from build123d import *

# Parameters (mm, degrees)
CHAMFER_1_SIZE      = 1
CUT_EXTRUDE_1_DEPTH = 37.221540553
SKETCH_3_R          = 10
EXTRUDE_1_DEPTH     = 15
CHAMFER_2_SIZE      = 0.5
SKETCH_7_W          = 0.7
SKETCH_7_H          = 1.1


with BuildPart() as part:
    # 草图1 → 旋转1 (revolve)
    with BuildSketch(Plane.XY, mode=Mode.PRIVATE) as revolve_1_sk:
        Polygon((0, 0), (10, 0), (10, 1.992934229), (10, 22), (12, 22), (12, 32), (9, 32), (9, 52), (0, 52), align=None)
    revolve(revolve_1_sk.sketch.rotate(Axis((0, 0, 0), (0, 1, 0)), 90), axis=Axis((0, 0, 0), (0, 1, 0)))

    # 倒角1
    chamfer_1_edges = [part.edges().sort_by_distance(p)[0] for p in [
        (0, 52, 9),
    ]]
    chamfer(chamfer_1_edges, length=CHAMFER_1_SIZE)

    # 草图2 → 切除-拉伸1 (cut, through all)
    with BuildSketch(Plane(origin=(0, 32, 0), x_dir=(1, 0, 0), z_dir=(0, 1, 0))):
        with BuildLine():
            Line((-11, -4.795831523), (-11, 4.795831523))
            ThreePointArc((-11, 4.795831523), (-12, 0), (-11, -4.795831523))
        make_face()
        with BuildLine():
            ThreePointArc((12, 0), (11.747340124, 2.449489743), (11, 4.795831523))
            Line((11, 4.795831523), (11, -4.795831523))
            ThreePointArc((11, -4.795831523), (11.747340124, -2.449489743), (12, 0))
        make_face()
    extrude(amount=-CUT_EXTRUDE_1_DEPTH, mode=Mode.SUBTRACT)

    # 草图3 → 凸台-拉伸1 (add)
    with BuildSketch(Plane.XZ):
        with Locations(Location((0, 0, 0), (0, 0, 270))):
            Circle(SKETCH_3_R)
    extrude(amount=EXTRUDE_1_DEPTH)

    # 倒角2
    chamfer_2_edges = [part.edges().sort_by_distance(p)[0] for p in [
        (0, -15, 10),
    ]]
    chamfer(chamfer_2_edges, length=CHAMFER_2_SIZE)

    # 草图7 → 切除-旋转1 (revolve, cut)
    with BuildSketch(Plane(origin=(0, 0, 0), x_dir=(0, 0, -1), z_dir=(1, 0, 0))):
        with Locations((9.65, -12.05)):
            Rectangle(SKETCH_7_W, SKETCH_7_H)
    revolve(axis=Axis((0, 52, 0), (0, -1, 0)), mode=Mode.SUBTRACT)


solid = part.part
Verification items for the finished model (mm, model axes). A direction names the side the tool comes from. Give positions to 0.01 mm unless a question says otherwise; leave off trailing zeros. Loops run counter-clockwise (first coordinate to the right, second up) from the corner with the lowest first, then second, coordinate; pieces in that order, holes last.
1) Thickness scan on line 1 along Y through (x, z) = (-9, -2.75); line 2 along Y through (x, z) = (3.5, -10); line 3 along Y through (x, z) = (7.5, -6.5). Record the ranges inside material, lowest first.
2) Depth check by flat-ended pin: pin 1 Ø6 at (x, y) = (5, 7.5) entering from -Z; pin 2 Ø2 at (x, y) = (1, 41.5) entering from -Z; pin 3 Ø1.5 at (x, y) = (-3, 13) entering from +Z. Enter the tip coordinate at first touch or a pass-through.
3) Set-up check for faces 1 (the cylindrical face through (-9.76, 5.48, 2.17)), 2 (the cylindrical face through (7.84, -12.04, -5)), 3 (the flat face through (-7, 32, 6)): record each of +Z, -Z, +X, -X, +Y, -Y from which the full face is reachable in a straight line by a thin tool's end or side.
4) Sectioned sample at D-D, the plane y = 5. Enter the section's corners in (x, z), then the cut area to 3 significant figures.
5) Sectioned sample at A-A, the plane z = 0. Enter the section's corners in (x, y), then the cut area to 3 significant figures.
6) Sectioned sample at B-B, the plane x = 0. Enter the section's corners in (y, z).
7) Sectioned sample at C-C, the plane y = 24. Enter the section's corners in (x, z), then the cut area to 3 significant figures.
8) Draft check along Y on faces 4 (the flat face through (-9, -12.6, 3)), 5 (the flat face through (11, 27, 0)), 6 (the flat face through (0, -15, 0)), 7 (the flat face through (-9, -11.5, 3)). Enter one of: pulls with the +Y half, pulls with the -Y half, needs draft (parallel to the pull), parting line crosses it, or undercut.
Answers:
1. line 1: y = -15 to -12.6, -11.5 to 32
1. line 2: y = 22 to 32
1. line 3: y = -14.58 to -12.6, -11.5 to 32
2. pin 1: stops at z = -9.8
2. pin 2: stops at z = -9
2. pin 3: stops at z = 9.74
3. face 1: -Y
3. face 2: none
3. face 3: +Y
4. outline: circle Ø20 at (0, 0)
4. area: 314 mm2
5. outline: (-11, 22) - (-10, 22) - (-10, -11.5) - (-9.3, -11.5) - (-9.3, -12.6) - (-10, -12.6) - (-10, -14.5) - (-9.5, -15) - (9.5, -15) - (10, -14.5) - (10, -12.6) - (9.3, -12.6) - (9.3, -11.5) - (10, -11.5) - (10, 22) - (11, 22) - (11, 32) - (9, 32) - (9, 51) - (8, 52) - (-8, 52) - (-9, 51) - (-9, 32) - (-11, 32) - close
5. area: 1,320 mm2
6. outline: (-15, -9.5) - (-14.5, -10) - (-12.6, -10) - (-12.6, -9.3) - (-11.5, -9.3) - (-11.5, -10) - (22, -10) - (22, -12) - (32, -12) - (32, -9) - (51, -9) - (52, -8) - (52, 8) - (51, 9) - (32, 9) - (32, 12) - (22, 12) - (22, 10) - (-11.5, 10) - (-11.5, 9.3) - (-12.6, 9.3) - (-12.6, 10) - (-14.5, 10) - (-15, 9.5) - close
7. outline: (-11, -4.8) arc R12 ccw to (11, -4.8) - (11, 4.8) arc R12 ccw to (-11, 4.8) - close
7. area: 439 mm2
8. face 4: undercut
8. face 5: needs draft
8. face 6: pulls with the -Y half
8. face 7: undercut
